Source: CAD feature listing. Evaluate the final solid. Frame: model axes, mm. Face numbers are marked on the shaded views. A direction names the side the tool comes from. Give positions to 0.01 mm unless a question says otherwise; leave off trailing zeros. Loops run counter-clockwise (first coordinate to the right, second up) from the corner with the lowest first, then second, coordinate; pieces in that order, holes last. Notation, with made-up numbers: M 27.25,62 L 56.25,62 A35 cw 56.25,96 Z; hole C 87,48.5 d3. An arc over 180 degrees is marked long. Put each result on its own line as item: value.
from build123d import *

# Parameters (mm, degrees)
SKETCH1_W           = 80.264
SKETCH1_H           = 158.75
BOSS_EXTRUDE1_DEPTH = 2.54
BOSS_EXTRUDE2_DEPTH = 25.4
FILLET1_R           = 7.62
SKETCH7_R           = 6.604
SKETCH7_R_2         = 9.525
SKETCH7_R_3         = 24.892
CUT_EXTRUDE1_DEPTH  = 181.068086556
BOSS_EXTRUDE3_DEPTH = 10.16


with BuildPart() as part:
    # Sketch1 → Boss-Extrude1 (new body)
    with BuildSketch(Plane(origin=(0, 0, 0), x_dir=(1, 0, 0), z_dir=(0, 1, 0))):
        with Locations((40.132, -79.375)):
            Rectangle(SKETCH1_W, SKETCH1_H)
    extrude(amount=BOSS_EXTRUDE1_DEPTH)

    # Sketch2 → Boss-Extrude2 (add)
    with BuildSketch(Plane(origin=(0, 2.54, 0), x_dir=(1, 0, 0), z_dir=(0, 1, 0))):
        with BuildLine():
            Line((3.81, -147.32), (3.81, -11.43))
            Line((3.81, -11.43), (3.81, 0))
            Line((3.81, 0), (0, 0))
            Line((0, 0), (0, -158.75))
            Line((0, -158.75), (80.264, -158.75))
            Line((80.264, -158.75), (80.264, 0))
            Line((80.264, 0), (76.454, 0))
            Line((76.454, 0), (76.454, -11.43))
            Line((76.454, -11.43), (76.454, -147.32))
            ThreePointArc((76.454, -147.32), (74.222153673, -152.708153673), (68.834, -154.94))
            Line((68.834, -154.94), (11.43, -154.94))
            ThreePointArc((11.43, -154.94), (6.041846327, -152.708153673), (3.81, -147.32))
        make_face()
    extrude(amount=BOSS_EXTRUDE2_DEPTH)

    # Fillet1
    fillet1_edges = [part.edges().sort_by_distance(p)[0] for p in [
        (0, 13.97, 0),
        (80.264, 13.97, 0),
        (80.264, 13.97, 158.75),
        (0, 13.97, 158.75),
    ]]
    fillet(fillet1_edges, radius=FILLET1_R)

    # Sketch7 → Cut-Extrude1 (cut, through all)
    with BuildSketch(Plane.XZ):
        with Locations(Location((40.132, 67.31, 0), (0, 0, 270))):
            Circle(SKETCH7_R)
        with Locations(Location((40.132, 100.6475, 0), (0, 0, 270))):
            Circle(SKETCH7_R_2)
        with Locations(Location((40.132, 30.48, 0), (0, 0, 270))):
            Circle(SKETCH7_R_3)
        with BuildLine():
            Line((40.64, 148.59), (12.7, 148.59))
            ThreePointArc((12.7, 148.59), (10.903948776, 147.846051224), (10.16, 146.05))
            Line((10.16, 146.05), (10.16, 118.11))
            ThreePointArc((10.16, 118.11), (10.903948776, 116.313948776), (12.7, 115.57))
            Line((12.7, 115.57), (40.64, 115.57))
            ThreePointArc((40.64, 115.57), (42.436051224, 116.313948776), (43.18, 118.11))
            Line((43.18, 118.11), (43.18, 146.05))
            ThreePointArc((43.18, 146.05), (42.436051224, 147.846051224), (40.64, 148.59))
        make_face()
    extrude(amount=-CUT_EXTRUDE1_DEPTH, mode=Mode.SUBTRACT)

    # Sketch8 → Boss-Extrude3 (add)
    with BuildSketch(Plane(origin=(80.264, 0, 0), x_dir=(0, 0, -1), z_dir=(1, 0, 0))):
        Polygon((-98.552, 27.94), (-101.6, 30.988), (-91.694, 30.988), (-94.742, 27.94), align=None)
        Polygon((-64.008, 27.94), (-60.198, 27.94), (-57.15, 30.988), (-67.056, 30.988), align=None)
        Polygon((-38.481, 30.988), (-35.433, 27.94), (-31.623, 27.94), (-28.575, 30.988), align=None)
    boss_extrude3 = extrude(amount=-BOSS_EXTRUDE3_DEPTH)

    # Mirror3: Boss-Extrude3 across plane
    add(boss_extrude3.mirror(Plane(origin=(40.132, 0, 0), x_dir=(0, 0, 1), z_dir=(1, 0, 0))))


solid = part.part
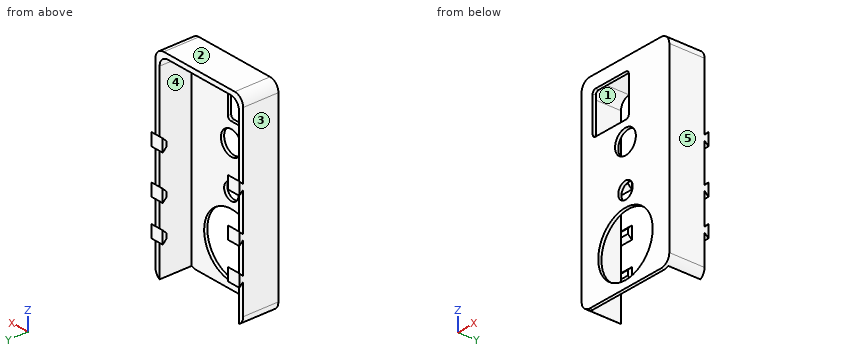
1. Access query for the marked faces 1 and 2. Directions: +Z, -Z, +X, -X, +Y, -Y. A direction counts if a zero-diameter tool reaches every point of the face in a straight line with its end or side. Return the directions, or none.
Found:
face 1: -Z, +Y
face 2: +Z, +X, -X, +Y, -Y
2. Contact query for flat-ended pins moving along their axis: P1, Ø2.5, axis at y = 29.5, z = 97, coming from the -X side; P2, Ø1, axis at x = 29, y = 12.5, coming from the -Z side; P3, Ø18, axis at x = 60, z = 133, coming from the +Y side; P4, Ø1.9, axis at x = 78.5, z = 16, coming from the +Y side. Output: stop coordinate, or through.
Found:
P1: x = 0
P2: z = 154.94
P3: y = 2.54
P4: y = 27.94
3. Draft query along X for the marked faces 3, 4 and 5. Return one class per face: pulls with the +X half, pulls with the -X half, needs draft (parallel to the pull), parting line crosses it, or undercut.
Found:
face 3: pulls with the -X half
face 4: undercut
face 5: pulls with the +X half
4. Section query A-A (x = 37). Output: boundary loops of the cut face in (y, z).
Found:
outline: M 0,0 L 2.54,0 L 2.54,5.79 L 0,5.79 Z; M 0,55.17 L 2.54,55.17 L 2.54,61.5 L 0,61.5 Z; M 0,73.12 L 2.54,73.12 L 2.54,91.65 L 0,91.65 Z; M 0,109.64 L 2.54,109.64 L 2.54,115.57 L 0,115.57 Z; M 0,148.59 L 2.54,148.59 L 2.54,154.94 L 27.94,154.94 L 27.94,158.75 L 0,158.75 Z
5. Material intervals for line 1 (X direction, y = 13.5, z = 103.5); line 2 (X direction, y = 29, z = 32.5); line 3 (Z direction, x = 71, y = 29), sorted ascending. Write a range as from..to.
Found:
line 1: 0..3.81, 76.45..80.26
line 2: 0..10.16, 70.1..80.26
line 3: 30.56..36.49, 59.14..65.07, 93.68..99.61
